Autodesk Inventor part; units mm, degrees
ref_plane "YZ Plane" through (0, 0, 0) normal (1, 0, 0) x (0, 1, 0)
ref_plane "XZ Plane" through (0, 0, 0) normal (0, 1, 0) x (-1, 0, 0)
ref_plane "XY Plane" through (0, 0, 0) normal (0, 0, 1) x (1, 0, 0)
sketch "Sketch1" plane through (0, 0, 0) normal (0, 1, 0) x (-1, 0, 0)
  line L0 (-31.75, 31.75) -> (31.75, 31.75)
  line L1 (31.75, 31.75) -> (31.75, -31.75)
  line L2 (31.75, -31.75) -> (-31.75, -31.75)
  line L3 (-31.75, -31.75) -> (-31.75, 31.75)
  line L4 (-31.75, 31.75) -> (31.75, -31.75) construction
  line L5 (31.75, 31.75) -> (-31.75, -31.75) construction
  point P0 (0, 0)
  dimension "d0" = 63.5
  dimension "d1" = 63.5
extrude "Extrusion1" add sketch "Sketch1" along normal blind 12.7
sketch "Sketch2" plane through (0, 12.7, 0) normal (0, 1, 0) x (1, 0, 0)
  line L0 (0, 0) -> (17.9605, 17.9605)
  line L1 (0, 0) -> (25.4, 0) construction
  line L2 (0, 0) -> (-17.9605, 17.9605)
  line L3 (0, 0) -> (-17.9605, -17.9605)
  line L4 (0, 0) -> (17.9605, -17.9605)
  dimension "d4" = 25.4
  dimension "d5" = 45
  dimension "d8" = 360
hole "Hole1" at (17.9605, 12.7, 17.9605) at (-17.9605, 12.7, -17.9605) at (-17.9605, 12.7, 17.9605) at (17.9605, 12.7, -17.9605) direction (0, -1, 0) diameter 6.7564 end up to surface counterbore diameter 19.05 counterbore depth 4.7752
sketch "Sketch3" plane through (0, 0, 0) normal (0, -1, 0) x (1, 0, 0)
  circle A0 centre (0, 0) radius 12.7
  dimension "d17" = 25.4
hole "Hole2" at (0, 0, 0) direction (0, 1, 0) diameter 6.7564 end up to surface counterbore diameter 19.05 counterbore depth 4.7752
properties part number "feet type 1 part 1" material "Stainless Steel"
CAD build for the part. Positions are in the model's coordinates, mm. A direction names the side the tool comes from. Coordinates: 2 decimals unless noted, no trailing zeros. Loops run counter-clockwise (first coordinate to the right, second up) from the corner with the lowest first, then second, coordinate; pieces in that order, holes last. Notation, with made-up numbers: (-18, 82.25) - (-8, 82.25) arc R19 cw to (-8, 113.25) - close; hole circle Ø2 at (0, 87). An arc over 180 degrees is marked (long way). Use one line per item in the form item = value. Start each with the question number.
1) Band-saw the part on A-A (z = 0). Give the cut face in (x, y) (3 decimals), and give its area (3 significant figures).
2) Band-saw the part on C-C (y = 4). State how many separate pieces and enclosed holes the cut face has, and give its area (3 significant figures).
3) Tool access for faces 1 (the face through (-31.75, 6, 0)), 2 (the face through (0, 4.775, -4)), 3 (the face through (18, 7.925, -14)): list every direction of +Z, -Z, +X, -X, +Y, -Y with a clear straight run to the whole face (end or side of a thin tool).
4) Band-saw the part on D-D (x = -19). Give the cut face in (y, z), and give its area (3 significant figures).
5) Flat gauge pins, fed straight in: pin 1 (11 mm diameter, centred on x = 17.96, z = -17.96, fed in from +Y); pin 2 (8 mm diameter, centred on x = 0, z = 0, fed in from -Y); pin 3 (4 mm diameter, centred on x = -17.96, z = -17.96, fed in from -Y). Where does each tip first touch, or does it go through?
6) Drill centre lines: L1, parallel to X at y = 9.5, z = -10.5; L2, parallel to X at y = 0.5, z = -17.5; L3, parallel to Z at x = 17, y = 7.75. Where is each one in solid material? Low to high. Write a range as from..to.
7) Band-saw the part on B-B (x = 0). Give the cut face in (y, z) (3 decimals).
8) Two-plate mould, pull along Z, no slides. Class faces 4 (the face through (17.542, 10.279, -27.476)), 5 (the face through (8, 12.7, 0)), 6 (the face through (0, 6, 31.75)), 7 (the face through (9.93, 10.28, 23.08)): +Z half, -Z half, draft (parallel to the pull), parting line (faces both ways), or undercut.
Check values:
q1.outline = (-31.75, 0) - (-9.525, 0) - (-9.525, 4.775) - (-3.378, 4.775) - (-3.378, 12.7) - (-31.75, 12.7) - close; (3.378, 4.775) - (9.525, 4.775) - (9.525, 0) - (31.75, 0) - (31.75, 12.7) - (3.378, 12.7) - close
q1.area = 662 mm2
q2.separate_pieces = 1
q2.enclosed_holes = 5
q2.area = 3,600 mm2
q3.face_1 = +Z, -Z, -X, +Y, -Y
q3.face_2 = -Y
q3.face_3 = +Y
q4.outline = (0, -31.75) - (12.7, -31.75) - (12.7, -27.43) - (7.92, -27.43) - (7.92, -21.17) - (0, -21.17) - close; (0, -14.75) - (7.92, -14.75) - (7.92, -8.49) - (12.7, -8.49) - (12.7, 8.49) - (7.92, 8.49) - (7.92, 14.75) - (0, 14.75) - close; (0, 21.17) - (7.92, 21.17) - (7.92, 27.43) - (12.7, 27.43) - (12.7, 31.75) - (0, 31.75) - close
q4.area = 524 mm2
q5.pin_1 = 7.92
q5.pin_2 = 4.78
q5.pin_3 = through
q6.L1 = -31.75..-23.88, -12.04..12.04, 23.88..31.75
q6.L2 = -31.75..-21.31, -14.61..14.61, 21.31..31.75
q6.L3 = -31.75..-21.2, -14.72..14.72, 21.2..31.75
q7.outline = (0, -31.75) - (12.7, -31.75) - (12.7, -3.378) - (4.775, -3.378) - (4.775, -9.525) - (0, -9.525) - close; (0, 9.525) - (4.775, 9.525) - (4.775, 3.378) - (12.7, 3.378) - (12.7, 31.75) - (0, 31.75) - close
q8.face_4 = undercut
q8.face_5 = draft
q8.face_6 = +Z half
q8.face_7 = undercut
